CAD build for the part. Positions are in the model's coordinates, mm. A direction names the side the tool comes from. Coordinates: 2 decimals unless noted, no trailing zeros. Loops run counter-clockwise (first coordinate to the right, second up) from the corner with the lowest first, then second, coordinate; pieces in that order, holes last. Notation, with made-up numbers: (11.5, 66.5) -> (43.5, 66.5) arc R18 cw to (43.5, 96.5) -> close; hole circle Ø4 at (-9, 5). An arc over 180 degrees is marked (long way). Write item = value, one per line. Start each with the question number.
(1) Band-saw the part on D-D (z = 1.5). Write the cut outline in (x, y), and give its area (3 significant figures).
(2) Band-saw the part on C-C (y = -13). Write the cut outline in (x, z), and give its area (3 significant figures).
(3) Pull direction X, two halves, no side cores. Call faces 4 (the face through (21, -14, 6)), 5 (the face through (30.4, -13.7, 0)), 6 (the face through (19, -14, 7)): +X half, -X half, draft (parallel to the pull), parting line (faces both ways), or undercut.
(4) Tool access for faces 1 (the face through (24, -17, 7)), 2 (the face through (24.549, -8.535, 7.301)), 3 (the face through (24.5, -12.25, 4.5)): list every direction of +Z, -Z, +X, -X, +Y, -Y with a clear straight run to the whole face (end or side of a thin tool).
(5) Flat gauge pins, fed straight in: P1, Ø1.6, axis at x = 24, y = -17.5, coming from the -Z side; P2, Ø0.9, axis at x = 24.5, z = 7, coming from the -Y side; P3, Ø4, axis at x = 25, y = -14, coming from the +Z side. Where does each tip first touch, or does it go through?
(6) Band-saw the part on B-B (x = 21.5). Count the separate pieces of the cut face and the enclosed holes in it, and give its area (3 significant figures).
(7) Drill centre lines: line 1 (Y direction, x = 15.5, z = 3.75); line 2 (Y direction, x = 21.5, z = 4.25); line 3 (X direction, y = -8.25, z = 1.25). Where is each one in solid material? Low to high. Write a range as from..to.
(8) Band-saw the part on A-A (z = 6). Write the cut outline in (x, y), and give its area (3 significant figures).
```python
from build123d import *

# Parameters (mm, degrees)
F0_W     = 30
F0_H     = 1
F1_DEPTH = 5
F2_DEPTH = 9
F3_DEPTH = 4
F4_W     = 3.5
F4_H     = 2
F5_DEPTH = 25
F6_R     = 0.99999


# Not quite as in the source:
# - a fillet or chamfer is up to 0.001 mm smaller than in the source, because OpenCascade refuses the exact size


with BuildPart() as f1:
    # F0 (on Top) → F1 (new body)
    with BuildSketch(Plane.XY):
        with Locations((15, -0.5)):
            Rectangle(F0_W, F0_H)
        Polygon((31, 0), (30, 0), (30, -1), (30, -8.25), (30, -13.75), (30, -19.25), (30, -26.5), (30, -27.5), (31, -27.5), align=None)
        with Locations((15, -27)):
            Rectangle(F0_W, F0_H)
        Polygon((30, -1), (0, -1), (0, -13.75), (19, -13.75), (19, -8.25), (30, -8.25), align=None)
        Polygon((19, -13.75), (0, -13.75), (0, -26.5), (30, -26.5), (30, -19.25), (19, -19.25), align=None)
    extrude(amount=F1_DEPTH)

    # F0 (on Top) → F2 (join)
    with BuildSketch(Plane.XY):
        Polygon((30, -13.75), (30, -8.25), (19, -8.25), (19, -13.75), (21, -13.75), (21, -12.25), (28, -12.25), (28, -13.75), align=None)
        Polygon((21, -13.75), (19, -13.75), (19, -19.25), (30, -19.25), (30, -13.75), (28, -13.75), (28, -15.25), (21, -15.25), align=None)
    extrude(amount=F2_DEPTH)

    # F0 (on Top) → F3 (cut)
    with BuildSketch(Plane.XY):
        Polygon((30, -1), (0, -1), (0, -13.75), (19, -13.75), (19, -8.25), (30, -8.25), align=None)
        Polygon((19, -13.75), (0, -13.75), (0, -26.5), (30, -26.5), (30, -19.25), (19, -19.25), align=None)
        Polygon((21, -13.75), (19, -13.75), (19, -19.25), (30, -19.25), (30, -13.75), (28, -13.75), (28, -15.25), (21, -15.25), align=None)
        Polygon((30, -13.75), (30, -8.25), (19, -8.25), (19, -13.75), (21, -13.75), (21, -12.25), (28, -12.25), (28, -13.75), align=None)
    extrude(amount=F3_DEPTH, mode=Mode.SUBTRACT)

    # F4 (on face) → F5 (cut)
    with BuildSketch(Plane(origin=(0, -8.25, 0), x_dir=(-1, 0, 0), z_dir=(0, 1, 0))):
        with Locations((-26.25, 6)):
            Rectangle(F4_W, F4_H)
        with Locations((-22.75, 6)):
            Rectangle(F4_W, F4_H)
    extrude(amount=-F5_DEPTH, mode=Mode.SUBTRACT)

    # F6 (radius 1 in the source; OpenCascade refuses exactly that, so slightly less here)
    f6_edges = [f1.edges().sort_by_distance(p)[0] for p in [
        (24.5, -19.25, 9),
        (24.5, -12.25, 9),
        (24.5, -12.25, 7),
        (24.5, -8.25, 9),
        (24.5, -15.25, 9),
        (24.5, -15.25, 7),
        (24.5, -19.25, 7),
        (24.5, -8.25, 7),
    ]]
    fillet(f6_edges, radius=F6_R)


solid = f1.part
```
Findings below:
q1.outline = (0, -27.5) -> (31, -27.5) -> (31, 0) -> (0, 0) -> (0, -1) -> (30, -1) -> (30, -26.5) -> (0, -26.5) -> close
q1.area = 87.5 mm²
q2.outline = (0, 4) -> (21, 4) -> (21, 9) -> (19, 9) -> (19, 5) -> (0, 5) -> close; (28, 4) -> (30, 4) -> (30, 0) -> (31, 0) -> (31, 5) -> (30, 5) -> (30, 9) -> (28, 9) -> close
q2.area = 44.0 mm²
q3.face_4 = undercut
q3.face_5 = draft
q3.face_6 = -X half
q4.face_1 = +Y, -Y
q4.face_2 = +Y
q4.face_3 = +Z, -Z
q5.P1 = 4
q5.P2 = -19.09
q5.P3 = 8.97
q6.separate_pieces = 4
q6.enclosed_holes = 0
q6.area = 46.8 mm²
q7.line_1 = -27.5..-26.5, -1..0
q7.line_2 = -27.5..-15.25, -12.25..0
q7.line_3 = 30..31
q8.outline = (19, -19.25) -> (21, -19.25) -> (21, -8.25) -> (19, -8.25) -> close; (28, -19.25) -> (30, -19.25) -> (30, -8.25) -> (28, -8.25) -> close
q8.area = 44.0 mm²
